Autodesk Inventor part; units mm, degrees
ref_plane "YZ Plane" through (0, 0, 0) normal (1, 0, 0) x (0, 1, 0)
ref_plane "XZ Plane" through (0, 0, 0) normal (0, 1, 0) x (-1, 0, 0)
ref_plane "XY Plane" through (0, 0, 0) normal (0, 0, 1) x (1, 0, 0)
sketch "Sketch1" plane through (0, 0, 0) normal (0, 0, 1) x (1, 0, 0)
  line L0 (135.5, -53.5) -> (140.5, -53.5)
  arc A0 (140.5, -56.5) -> (140.5, -53.5) centre (140.5, -55) ccw
  line L1 (140.5, -56.5) -> (135.5, -56.5)
  arc A1 (135.5, -53.5) -> (135.5, -56.5) centre (135.5, -55) ccw
  line L2 (30.5, -21.5) -> (35.5, -21.5)
  arc A2 (35.5, -24.5) -> (35.5, -21.5) centre (35.5, -23) ccw
  line L3 (35.5, -24.5) -> (30.5, -24.5)
  arc A3 (30.5, -21.5) -> (30.5, -24.5) centre (30.5, -23) ccw
  line L4 (35.5, -56.5) -> (30.5, -56.5)
  arc A4 (30.5, -53.5) -> (30.5, -56.5) centre (30.5, -55) ccw
  line L5 (30.5, -53.5) -> (35.5, -53.5)
  arc A5 (35.5, -56.5) -> (35.5, -53.5) centre (35.5, -55) ccw
  line L6 (140.5, -24.5) -> (135.5, -24.5)
  arc A6 (135.5, -21.5) -> (135.5, -24.5) centre (135.5, -23) ccw
  line L7 (135.5, -21.5) -> (140.5, -21.5)
  arc A7 (140.5, -24.5) -> (140.5, -21.5) centre (140.5, -23) ccw
  arc A8 (6.0006, -22.6082) -> (8.7763, -25.5998) centre (9.0006, -22.6082) ccw
  line L8 (8.7763, -25.5998) -> (27.4457, -27)
  arc A9 (27.2213, -26.9916) -> (27.4457, -27) centre (27.4457, -24) ccw
  line L9 (27.4457, -27) -> (80, -27)
  arc A10 (83, -30) -> (80, -27) centre (80, -30) ccw
  line L10 (83, -30) -> (83, -48.0084)
  arc A11 (80, -51.0084) -> (83, -48.0084) centre (80, -48.0084) ccw
  line L11 (80, -51.0084) -> (27.2213, -51.0084)
  arc A12 (27.4457, -51) -> (27.2213, -51.0084) centre (27.4457, -54) ccw
  line L12 (27.2213, -51.0084) -> (8.7756, -52.3918)
  arc A13 (8.7756, -52.3918) -> (6, -55.3834) centre (9, -55.3834) ccw
  line L13 (6, -55.3834) -> (6, -64)
  arc A14 (6, -64) -> (14, -64) centre (10, -64) ccw
  line L14 (14, -64) -> (14, -62)
  arc A15 (17, -59) -> (14, -62) centre (17, -62) ccw
  line L15 (17, -59) -> (78, -59)
  arc A16 (81, -62) -> (78, -59) centre (78, -62) ccw
  line L16 (81, -62) -> (81, -64)
  arc A17 (81, -64) -> (89, -64) centre (85, -64) ccw
  line L17 (89, -64) -> (89, -62)
  arc A18 (92, -59) -> (89, -62) centre (92, -62) ccw
  line L18 (92, -59) -> (152.9994, -59)
  arc A19 (155.9994, -62) -> (152.9994, -59) centre (152.9994, -62) ccw
  line L19 (155.9994, -62) -> (155.9994, -64)
  arc A20 (155.9994, -64) -> (163.9994, -64) centre (159.9994, -64) ccw
  line L20 (163.9994, -64) -> (163.9994, -55.3918)
  arc A21 (163.9994, -55.3918) -> (161.2237, -52.4002) centre (160.9994, -55.3918) ccw
  line L21 (161.2237, -52.4002) -> (142.5543, -51)
  arc A22 (142.7787, -51.0084) -> (142.5543, -51) centre (142.5543, -54) ccw
  line L22 (142.5543, -51) -> (106, -51)
  arc A23 (103, -48) -> (106, -51) centre (106, -48) ccw
  line L23 (103, -48) -> (103, -29.9916)
  arc A24 (106, -26.9916) -> (103, -29.9916) centre (106, -29.9916) ccw
  line L24 (106, -26.9916) -> (142.7787, -26.9916)
  arc A25 (142.5543, -27) -> (142.7787, -26.9916) centre (142.5543, -24) ccw
  line L25 (142.7787, -26.9916) -> (161.2244, -25.6082)
  arc A26 (161.2244, -25.6082) -> (164.0006, -22.6166) centre (161.0006, -22.6165) ccw
  line L26 (164.0006, -22.6166) -> (164.0006, -14)
  arc A27 (164.0006, -14) -> (156.0006, -14) centre (160.0006, -14) ccw
  line L27 (156.0006, -14) -> (156.0006, -16)
  arc A28 (153.0006, -19) -> (156.0006, -16) centre (153.0006, -16) ccw
  line L28 (153.0006, -19) -> (92.0006, -19)
  arc A29 (89.0006, -16) -> (92.0006, -19) centre (92.0006, -16) ccw
  line L29 (89.0006, -16) -> (89.0006, -14)
  arc A30 (89.0006, -14) -> (81.0006, -14) centre (85.0006, -14) ccw
  line L30 (81.0006, -14) -> (81.0006, -16)
  arc A31 (78.0006, -19) -> (81.0006, -16) centre (78.0006, -16) ccw
  line L31 (78.0006, -19) -> (17.0006, -19)
  arc A32 (14.0006, -16) -> (17.0006, -19) centre (17.0006, -16) ccw
  line L32 (14.0006, -16) -> (14.0006, -14)
  arc A33 (14.0006, -14) -> (6.0006, -14) centre (10.0006, -14) ccw
  line L33 (6.0006, -14) -> (6.0006, -22.6082)
  arc A34 (98, -37) -> (88, -37) centre (93, -37) ccw
  line L34 (98, -37) -> (98, -41)
  arc A35 (88, -41) -> (98, -41) centre (93, -41) ccw
  line L35 (88, -41) -> (88, -37)
  circle A36 centre (10, -14) radius 1.5
  circle A37 centre (10, -64) radius 1.5
  circle A38 centre (85, -64) radius 1.5
  circle A39 centre (85, -14) radius 1.5
  circle A40 centre (160, -14) radius 1.5
  circle A41 centre (160, -64) radius 1.5
  point P0 (0, 0)
extrude "Extrusion1" add sketch "Sketch1" along normal blind 3
properties part number "updown_slider"
Verification items for the finished model (mm, model axes). A direction names the side the tool comes from. Coordinates: 2 decimals unless noted, no trailing zeros. Order: outer loops, then holes, each group sorted by start corner. A loop starts at its lowest first (then second) coordinate and runs counter-clockwise, first axis right, second up. Notation, with made-up numbers: (15.5, -28) -> (69.5, -28) arc R17 ccw to (69.5, -7) -> close; hole circle Ø5 at (-36, -36.5). An arc over 180 degrees is marked (long way). Put each result on its own line as item: value. Start each with the question number.
1) Material ranges on L1, parallel to Y at x = 77.5, z = 0.5; L2, parallel to Y at x = 85, z = 0.85; L3, parallel to X at y = -17.5, z = 2.05, recorded low to high.
2) Cross-section at A-A (x = 34). Enter the section's corners in (y, z).
3) Cross-section at B-B (x = 119). Enter the section's corners in (y, z), plus the area to 3 significant figures.
4) Go/stop test with flat-tipped pins: pin 1 (0.9 mm diameter, centred on x = 138, z = 1, fed in from +Y); pin 2 (1.5 mm diameter, centred on y = -41, z = 2, fed in from +X); pin 3 (1.5 mm diameter, centred on y = -39.5, z = 2, fed in from -X); pin 4 (1.8 mm diameter, centred on x = 160, y = -64, fed in from +Z). Record where each tip stops, or that it passes through.
5) Tool access check on faces 1 (the flat face through (48, -19, 1)), 2 (the flat face through (152.02, -51.71, 1.48)), 3 (the cylindrical face through (14.86, -59.9, 1.48)), 4 (the cylindrical face through (142, -55, 1)). Record the directions out of +Z, -Z, +X, -X, +Y, -Y that give a thin tool (end or side, any length) a straight path to the whole face; none if there is none.
6) Release check for a two-part mould opening along X. For faces 5 (the cylindrical face through (8.5, -14.07, 1.48)), 6 (the flat face through (163.999, -60, 1)), 7 (the cylindrical face through (85, -10, 1)), 8 (the flat face through (124, -26.992, 1)) record: pulls with the +X half, pulls with the -X half, needs draft (parallel to the pull), parting line crosses it, or undercut.
7) Cross-section at C-C (z = 2). State how many separate pieces and enclosed holes the cut face has, plus the area to 3 significant figures.
Geometry check:
1. L1: y = -59 to -51.01, -27 to -19
1. L2: y = -68 to -65.5, -62.5 to -15.5, -12.5 to -10
1. L3: x = 6 to 14.4, 80.6 to 89.4, 155.6 to 164
2. outline: (-59, 0) -> (-56.5, 0) -> (-56.5, 3) -> (-59, 3) -> close; (-53.5, 0) -> (-51.01, 0) -> (-51.01, 3) -> (-53.5, 3) -> close; (-27, 0) -> (-24.5, 0) -> (-24.5, 3) -> (-27, 3) -> close; (-21.5, 0) -> (-19, 0) -> (-19, 3) -> (-21.5, 3) -> close
3. outline: (-59, 0) -> (-51, 0) -> (-51, 3) -> (-59, 3) -> close; (-26.99, 0) -> (-19, 0) -> (-19, 3) -> (-26.99, 3) -> close
3. area: 48.0 mm^2
4. pin 1: stops at y = -19
4. pin 2: stops at x = 103
4. pin 3: stops at x = 83
4. pin 4: passes through
5. face 1: +Z, -Z, +Y
5. face 2: +Z, -Z, +X
5. face 3: +Z, -Z, -Y
5. face 4: +Z, -Z
6. face 5: undercut
6. face 6: pulls with the +X half
6. face 7: undercut
6. face 8: needs draft
7. separate pieces: 1
7. enclosed holes: 11
7. area: 3,100 mm^2
